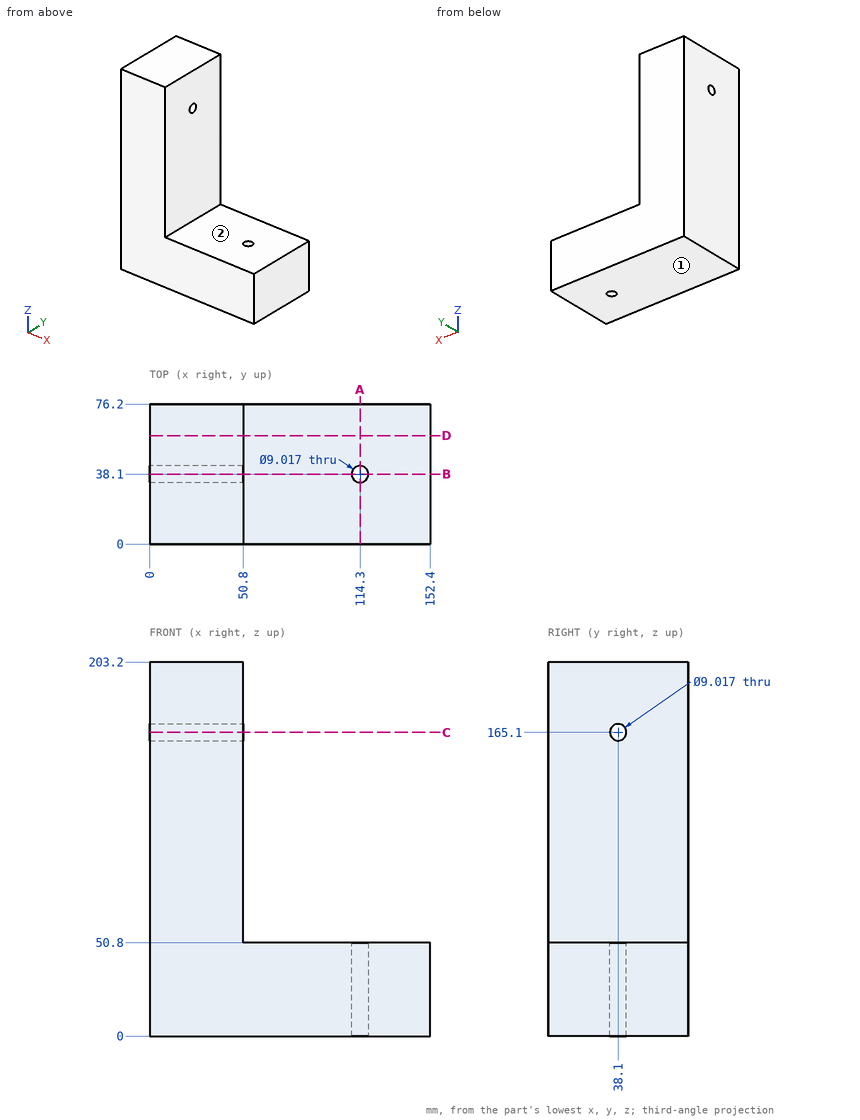
Geometry check sheet. Reference: drawing and pictorial views, mm from the part's lowest x, y, z. A direction names the side the tool comes from. Round coordinates to 2 decimals unless told otherwise and drop trailing zeros. Order: outer loops, then holes, each group sorted by start corner. A loop starts at its lowest first (then second) coordinate and runs counter-clockwise, first axis right, second up.
Q1. Depth check by flat-ended pin: P1, Ø23, axis at x = 101.5, y = 41, coming from the +Z side; P2, Ø6, axis at y = 65, z = 94.5, coming from the +X side. Enter the tip coordinate at first touch or a pass-through.
Filled sheet:
P1: stops at z = 50.8
P2: stops at x = 50.8
Q2. Scan lines: L1, parallel to X at y = 38, z = 12; L2, parallel to Y at x = 27.5, z = 165; L3, parallel to Z at x = 24.5, y = 38. Record each from-to range of solid material in increasing order.
Filled sheet:
L1: x = 0 to 109.79, 118.81 to 152.4
L2: y = 0 to 33.59, 42.61 to 76.2
L3: z = 0 to 160.59, 169.61 to 203.2
Q3. Cross-section at A-A, the plane x = 114.3. Enter the section's corners in (y, z), plus the area to 3 significant figures.
Filled sheet:
outline: (0, 0) - (33.59, 0) - (33.59, 50.8) - (0, 50.8) - close; (42.61, 0) - (76.2, 0) - (76.2, 50.8) - (42.61, 50.8) - close
area: 3,410 mm2
Q4. Cross-section at C-C, the plane z = 165.1. Enter the section's corners in (x, y).
Filled sheet:
outline: (0, 0) - (50.8, 0) - (50.8, 33.59) - (0, 33.59) - close; (0, 42.61) - (50.8, 42.61) - (50.8, 76.2) - (0, 76.2) - close
Q5. Cross-section at D-D, the plane y = 59. Enter the section's corners in (x, z), plus the area to 3 significant figures.
Filled sheet:
outline: (0, 0) - (152.4, 0) - (152.4, 50.8) - (50.8, 50.8) - (50.8, 203.2) - (0, 203.2) - close
area: 15,500 mm2
Q6. Set-up check for the marked faces 1 and 2: record each of +Z, -Z, +X, -X, +Y, -Y from which the full face is reachable in a straight line by a thin tool's end or side.
Filled sheet:
face 1: -Z, +X, -X, +Y, -Y
face 2: +Z, +X, +Y, -Y
Q7. Cross-section at B-B, the plane y = 38.1. Enter the section's corners in (x, z).
Filled sheet:
outline: (0, 0) - (109.79, 0) - (109.79, 50.8) - (50.8, 50.8) - (50.8, 160.59) - (0, 160.59) - close; (0, 169.61) - (50.8, 169.61) - (50.8, 203.2) - (0, 203.2) - close; (118.81, 0) - (152.4, 0) - (152.4, 50.8) - (118.81, 50.8) - close
